from build123d import *

# Parameters (mm, degrees)
BOSS_EXTRUDE1_DEPTH = 66.1
BOSS_EXTRUDE2_DEPTH = 3.05
BOSS_EXTRUDE3_DEPTH = 3.175
SKETCH2_4_R         = 1.5
CUT_EXTRUDE1_DEPTH  = 3
CHAMFER1_SIZE       = 1.5
CHAMFER3_SIZE       = 3.175


with BuildPart() as part:
    # Sketch1 → Boss-Extrude1 (new body)
    with BuildSketch(Plane(origin=(0, 0, 0), x_dir=(0, 0, -1), z_dir=(1, 0, 0))):
        Polygon((14.702260095, 19.28355698), (34.702260095, 19.28355698), (34.702260095, 0), (0, 0), (0, 19.28355698), (10, 19.28355698), (24.28355698, 5), (26.634687027, 7.351130047), align=None)
    extrude(amount=BOSS_EXTRUDE1_DEPTH)

    # Sketch1<4> → Boss-Extrude2 (add)
    with BuildSketch(Plane(origin=(0, 0, 0), x_dir=(0, 0, -1), z_dir=(1, 0, 0))):
        Polygon((23.806259903, 10.179557172), (21.455129855, 7.828427125), (24.28355698, 5), (26.634687027, 7.351130047), align=None)
    boss_extrude2 = extrude(amount=BOSS_EXTRUDE2_DEPTH)

    # Mirror1: Boss-Extrude2 across plane
    add(boss_extrude2.mirror(Plane.ZY.offset(-33.05)))

    # Sketch2 → Boss-Extrude3 (add)
    with BuildSketch(Plane(origin=(0, 0, 0), x_dir=(1, 0, 0), z_dir=(0, 1, 0))):
        Polygon((0, 11.276130047), (0, 0), (66.1, 0), (66.1, 11.276130047), (63.1, 11.276130047), (63.1, 7.176130047), (3, 7.176130047), (3, 11.276130047), align=None)
        Polygon((0, 34.702260095), (0, 19.376130047), (3, 19.376130047), (3, 27.526130047), (63.1, 27.526130047), (63.1, 19.376130047), (66.1, 19.376130047), (66.1, 34.702260095), align=None)
    extrude(amount=-BOSS_EXTRUDE3_DEPTH)

    # Sketch2<4> → Cut-Extrude1 (cut)
    with BuildSketch(Plane(origin=(0, 0, 0), x_dir=(1, 0, 0), z_dir=(0, 1, 0))):
        with Locations(Location((54.05, 14.176130047, 0), (0, 0, 90))):
            Circle(SKETCH2_4_R)
        with Locations(Location((12.05, 14.176130047, 0), (0, 0, 90))):
            Circle(SKETCH2_4_R)
    extrude(amount=CUT_EXTRUDE1_DEPTH, mode=Mode.SUBTRACT)

    # Chamfer1
    chamfer1_edges = [part.edges().sort_by_distance(p)[0] for p in [
        (54.05, 3, -12.676130047),
        (54.05, 0, -12.676130047),
        (12.05, 0, -12.676130047),
        (12.05, 3, -12.676130047),
    ]]
    chamfer(chamfer1_edges, length=CHAMFER1_SIZE - 0.0001)  # a hair under: the kernel refuses the full size

    # Chamfer3
    chamfer3_edges = [part.edges().sort_by_distance(p)[0] for p in [
        (33.05, 0, -27.526130047),
    ]]
    chamfer(chamfer3_edges, length=CHAMFER3_SIZE - 0.0001)  # a hair under: the kernel refuses the full size


solid = part.part
Part model, mm, in its own coordinate system. A direction names the side the tool comes from. Coordinates: 2 decimals unless noted, no trailing zeros. Loops run counter-clockwise (first coordinate to the right, second up) from the corner with the lowest first, then second, coordinate; pieces in that order, holes last. Notation, with made-up numbers: M 3,45.5 L 8,45.5 A29 ccw 8,79.5 Z; hole C 72.25,36 d5. An arc over 180 degrees is marked long. Use a Markdown table: item, result. Add a question column.
Q1. Cut at D-D (y = 16). Write the cut outline in (x, z), and give its area (3 significant figures).
Q2. Pin check, flat tip, straight feed: P1, Ø5, axis at x = 12.05, z = -14.18, coming from the -Y side. Stop position of the tip, or through.
Q3. Cut at A-A (y = -2). Write the cut outline in (x, z), and give its area (3 significant figures).
Q4. Probe L1, parallel to X at y = 6, z = -25; L2, parallel to Z at x = 54.05, y = 1.5; L3, parallel to Y at x = 43.5, z = -8. List the from-to ranges inside material, lowest first.
Q5. Mould opens along X. For faces 5 (the flat face through (63.1, -2, -9)), 6 (the flat face through (33, 8, 0)), 7 (the flat face through (0, 8, -18)) say: +X half, -X half, draft (parallel to the pull), parting line (faces both ways), or undercut.
Q6. Which spindle directions (+Z, -Z, +X, -X, +Y, -Y) get a long thin tool onto all of the face, cutting with end or side? Do faces 1 (the flat face through (3, -2, -22)), 2 (the flat face through (1.504, 9.02, -22.647)), 3 (the flat face through (63.05, 8, -24)), 4 (the flat face through (1, -2, -19.376)). Say none if no direction does.
Q7. Cut at C-C (y = 6.25). Write the cut outline in (x, z).
Worked out:
| question | item | result |
|---|---|---|
| 1 | outline | M 0,-34.7 L 66.1,-34.7 L 66.1,-17.99 L 0,-17.99 Z; M 0,-13.28 L 66.1,-13.28 L 66.1,0 L 0,0 Z |
| 1 | area | 1,980 mm2 |
| 2 | P1 | stops at y = 0.5 |
| 3 | outline | M 0,-34.7 L 66.1,-34.7 L 66.1,-19.38 L 63.1,-19.38 L 63.1,-26.35 L 3,-26.35 L 3,-19.38 L 0,-19.38 Z; M 0,-11.28 L 3,-11.28 L 3,-7.18 L 63.1,-7.18 L 63.1,-11.28 L 66.1,-11.28 L 66.1,0 L 0,0 Z |
| 3 | area | 1,090 mm2 |
| 4 | L1 | x = 0 to 3.05, 63.05 to 66.1 |
| 4 | L2 | z = -34.7 to -15.68, -12.68 to 0 |
| 4 | L3 | y = 0 to 19.28 |
| 5 | face 5 | undercut |
| 5 | face 6 | draft |
| 5 | face 7 | -X half |
| 6 | face 1 | -Y |
| 6 | face 2 | +X, -X |
| 6 | face 3 | none |
| 6 | face 4 | +X, -X, -Y |
| 7 | outline | M 0,-34.7 L 66.1,-34.7 L 66.1,0 L 0,0 Z; hole M 3.05,-25.53 L 63.05,-25.53 L 63.05,-23.03 L 3.05,-23.03 Z |
